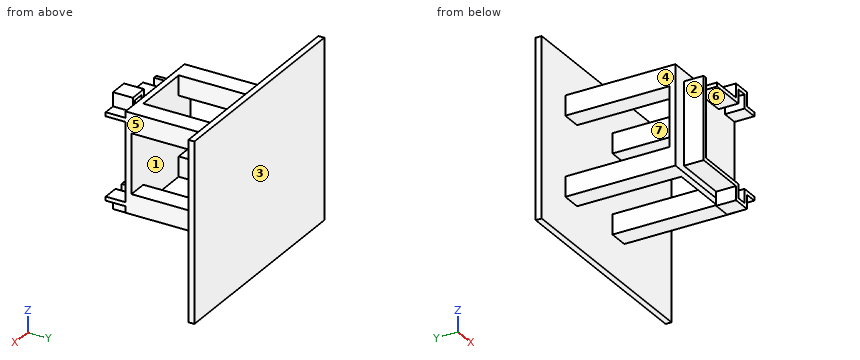
Autodesk Inventor part; units mm, degrees
ref_plane "YZ Plane" through (0, 0, 0) normal (1, 0, 0) x (0, 1, 0)
ref_plane "XZ Plane" through (0, 0, 0) normal (0, 1, 0) x (-1, 0, 0)
ref_plane "XY Plane" through (0, 0, 0) normal (0, 0, 1) x (1, 0, 0)
sketch "Sketch1" plane through (0, 0, 0) normal (0, 1, 0) x (-1, 0, 0)
  line L0 (25, 25) -> (15, 25)
  line L1 (15, 25) -> (15, 15)
  line L2 (15, 15) -> (25, 15)
  line L3 (25, 15) -> (25, 25)
  line L4 (25, 25) -> (-25, 25)
  line L5 (-25, 25) -> (-25, -25)
  line L6 (-25, -25) -> (25, -25)
  line L7 (25, -25) -> (25, 25)
  line L8 (25, 0) -> (-25, 0)
  line L9 (0, 25) -> (0, -25)
  line L10 (-25, 25) -> (-25, 15)
  line L11 (-15, 25) -> (-25, 25)
  line L12 (-15, 15) -> (-15, 25)
  line L13 (-25, 15) -> (-15, 15)
  line L14 (15, -15) -> (15, -25)
  line L15 (25, -15) -> (15, -15)
  line L16 (25, -25) -> (25, -15)
  line L17 (15, -25) -> (25, -25)
  line L18 (-25, -15) -> (-25, -25)
  line L19 (-15, -15) -> (-25, -15)
  line L20 (-15, -25) -> (-15, -15)
  line L21 (-25, -25) -> (-15, -25)
  line L22 (45, 45) -> (-45, 45)
  line L23 (-45, 45) -> (-45, -45)
  line L24 (-45, -45) -> (45, -45)
  line L25 (45, -45) -> (45, 45)
  point P0 (0, 0)
  point P1 (20, 25)
  point P2 (-20, 25)
  point P3 (20, -15)
  point P4 (-20, -15)
  point P5 (0, 45)
  dimension "d0" = 10
  dimension "d1" = 10
  dimension "d2" = 0
  dimension "d3" = 0
  dimension "d4" = 0
  dimension "d5" = 0
  dimension "d8" = 40
  dimension "d11" = 40
  dimension "d14" = 50
  dimension "d15" = 50
  dimension "d42" = 20
  dimension "d43" = 20
  dimension "d44" = 20
  dimension "d45" = 20
extrude "Extrusion1" add sketch "Sketch1" along normal blind 3 contours L1 L2 L7 L8 L9 L4 | L9 L8 L5 L13 L12 L4 | L7 L15 L14 L6 L9 L8 | L9 L6 L20 L19 L5 L8
extrude "Extrusion2" add sketch "Sketch1" along normal blind 55.594 contours L3 L2 L1 L0 | L12 L13 L5 L4 | L7 L6 L14 L15 | L19 L20 L6 L5
sketch "Sketch2" plane through (0, 0, 0) normal (0, -1, 0) x (1, 0, 0)
  line L0 (25, 15) -> (25, -15)
  line L1 (25, -19.8) -> (-15.893, -19.8)
  line L2 (-15.893, -19.8) -> (-15.893, 19.8)
  line L3 (-15.893, 19.8) -> (25, 19.8)
  line L4 (25, 19.8) -> (25, -19.8)
  line L5 (16.82, -19.8) -> (11.514, -19.8)
  line L6 (11.514, -19.8) -> (11.514, -26.8)
  line L7 (11.514, -26.8) -> (16.82, -26.8)
  line L8 (16.82, -26.8) -> (16.82, -19.8)
  line L9 (-15.893, 0) -> (25, 0)
  line L10 (11.514, 19.8) -> (11.514, 26.8)
  line L11 (11.514, 26.8) -> (16.82, 26.8)
  line L12 (16.82, 26.8) -> (16.82, 19.8)
  line L13 (-9.486, 19.8) -> (-5.486, 19.8)
  line L14 (9.514, 21.8) -> (-6.486, 21.8)
  line L15 (9.514, 21.8) -> (9.514, 28.8)
  line L16 (9.514, 28.8) -> (18.82, 28.8)
  line L17 (18.82, 28.8) -> (18.82, 21.8)
  line L18 (18.82, 21.8) -> (25, 21.8)
  line L19 (25, -15) -> (25, -25)
  line L20 (25, -21.8) -> (18.82, -21.8)
  line L21 (18.82, -21.8) -> (18.82, -28.8)
  line L22 (18.82, -28.8) -> (9.514, -28.8)
  line L23 (9.514, -28.8) -> (9.514, -21.8)
  line L24 (9.514, -21.8) -> (1.695, -21.8)
  line L25 (1.695, -21.8) -> (-17.893, -21.8)
  line L26 (-17.893, -21.8) -> (-17.893, 21.8)
  line L27 (25, 19.8) -> (25, 21.8)
  line L28 (25, -15) -> (25, -19.8)
  line L29 (25, -21.8) -> (25, -15)
  line L30 (-15.893, 19.8) -> (-17.893, 19.8)
  line L31 (-6.486, 21.8) -> (-6.486, 19.8)
  point P0 (0, 0)
  point P1 (16.82, -23.3)
  point P2 (4.5535, -19.8)
  point P3 (18.82, -25.3)
  point P4 (14.167, 28.8)
  point P5 (14.167, 26.8)
  point P6 (11.514, 23.3)
  point P7 (16.82, 19.8)
  point P8 (25, 14.5)
  point P9 (11.514, 19.8)
  point P10 (11.514, -19.8)
  point P11 (14.167, -28.8)
  dimension "d20" = 39.6
  dimension "d22" = 40.893
  dimension "d23" = 8.18
  dimension "d25" = 5.306
  dimension "d26" = 7
  dimension "d30" = 2
  dimension "d31" = 2
  dimension "d32" = 2
  dimension "d33" = 2
  dimension "d36" = 2
  dimension "d37" = 2
  dimension "d38" = 2
  dimension "d53" = 0
  dimension "d54" = 16
  dimension "d55" = 2
  dimension "d56" = 2
extrude "Extrusion3" add sketch "Sketch2" along normal blind 10 contours L3 L12 L11 L10 L31 L14 L15 L16 L17 L18 L27 | L2 L1 L6 L7 L8 L19 L20 L21 L22 L23 L24 L25 L26 L30
sketch "Sketch3" plane through (0, 55.594, 0) normal (0, 1, 0) x (1, 0, 0)
  line L0 (-45, -45) -> (65, -45)
  line L1 (65, -45) -> (65, 45)
  line L2 (65, 45) -> (-45, 45)
  line L3 (-45, 45) -> (-45, -45)
  line L4 (-25, -25) -> (-15, -25)
  line L5 (25, -25) -> (25, -15)
  line L6 (15, 25) -> (-15, 25)
  line L7 (-25, 15) -> (-25, -15)
  point P0 (0, 0)
  dimension "d46" = 20
  dimension "d47" = 40
  dimension "d48" = 20
  dimension "d49" = 20
extrude "Extrusion4" add sketch "Sketch3" along normal blind 3
properties part number "pitchrollmount44"
Model file for the job. Use its own axes, mm. Face numbers are marked on the shaded views. A direction names the side the tool comes from. Round coordinates to 2 decimals unless told otherwise and drop trailing zeros. Loops run counter-clockwise (first coordinate to the right, second up) from the corner with the lowest first, then second, coordinate; pieces in that order, holes last.
1. Band-saw the part on D-D, the plane y = 29. List the corners of the cut face in (x, z), and give its area (3 significant figures).
Check values:
outline: (-25, -25) - (-15, -25) - (-15, -15) - (-25, -15) - close; (-25, 15) - (-15, 15) - (-15, 25) - (-25, 25) - close; (15, -25) - (25, -25) - (25, -15) - (15, -15) - close; (15, 15) - (25, 15) - (25, 25) - (15, 25) - close
area: 400 mm2
2. Drop flat-ended pins along their axis: P1, Ø6, axis at x = 14.5, y = -4, coming from the +Z side; P2, Ø3.5, axis at y = -6, z = 24.5, coming from the -X side; P3, Ø1.5, axis at y = 2, z = 17.5, coming from the -X side. Give the stop position or say it passes through.
Check values:
P1: stops at z = 28.8
P2: stops at x = 9.51
P3: stops at x = -25
3. Mould opens along X. For the marked faces 1, 2 and 3 say: +X half, -X half, draft (parallel to the pull), parting line (faces both ways), or undercut.
Check values:
face 1: undercut
face 2: -X half
face 3: draft
4. Band-saw the part on B-B, the plane y = -3. List the corners of the cut face in (x, z), and give its area (3 significant figures).
Check values:
outline: (-17.89, -21.8) - (9.51, -21.8) - (9.51, -28.8) - (18.82, -28.8) - (18.82, -21.8) - (25, -21.8) - (25, -19.8) - (16.82, -19.8) - (16.82, -26.8) - (11.51, -26.8) - (11.51, -19.8) - (-15.89, -19.8) - (-15.89, 19.8) - (-17.89, 19.8) - close; (-6.49, 19.8) - (11.51, 19.8) - (11.51, 26.8) - (16.82, 26.8) - (16.82, 19.8) - (25, 19.8) - (25, 21.8) - (18.82, 21.8) - (18.82, 28.8) - (9.51, 28.8) - (9.51, 21.8) - (-6.49, 21.8) - close
area: 284 mm2
5. Band-saw the part on A-A, the plane x = -12.5. List the corners of the cut face in (y, z), and give its area (3 significant figures).
Check values:
outline: (-10, -21.8) - (0, -21.8) - (0, -25) - (3, -25) - (3, 25) - (0, 25) - (0, -19.8) - (-10, -19.8) - close; (55.59, -45) - (58.59, -45) - (58.59, 45) - (55.59, 45) - close
area: 440 mm2
6. Band-saw the part on C-C, the plane z = 3. List the corners of the cut face in (x, y).
Check values:
outline: (-45, 55.59) - (65, 55.59) - (65, 58.59) - (-45, 58.59) - close; (-25, 0) - (-17.89, 0) - (-17.89, -10) - (-15.89, -10) - (-15.89, 0) - (25, 0) - (25, 3) - (-25, 3) - close
7. Tool access for the marked faces 4, 5, 6 and 7: list every direction of +Z, -Z, +X, -X, +Y, -Y with a clear straight run to the whole face (end or side of a thin tool).
Check values:
face 4: +Z, -Z, -X, -Y
face 5: +Z, -Z, +X, -Y
face 6: +X, -Y
face 7: +Z, -Z
8. Wall check: probe 1 along X at (y, z) = (53, -22); probe 2 along Y at (x, z) = (3.5, -2.5). Give the ranges that are in metal, low to high.
Check values:
probe 1: x = -25 to -15, 15 to 25
probe 2: y = 0 to 3, 55.59 to 58.59
